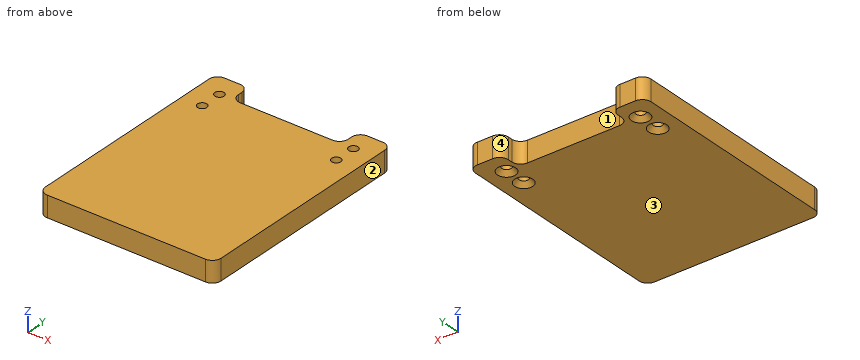
from build123d import *

# Parameters (mm, degrees)
F0_R     = 2.1
F1_DEPTH = 9.525
F2_SIZE2 = 2
F2_SIZE  = 2
F3_W     = 50
F3_H     = 10
F4_DEPTH = 25
F5_R     = 4
F6_R     = 4


with BuildPart() as f1:
    # F0 (on Top) → F1 (new body)
    with BuildSketch(Plane.XY):
        with BuildLine():
            ThreePointArc((40, 47.5), (38.8284271247, 50.3284271247), (36, 51.5))
            Line((36, 51.5), (-36, 51.5))
            ThreePointArc((-36, 51.5), (-38.8284271247, 50.3284271247), (-40, 47.5))
            Line((-40, 47.5), (-40, -47.5))
            ThreePointArc((-40, -47.5), (-38.8284271247, -50.3284271247), (-36, -51.5))
            Line((-36, -51.5), (36, -51.5))
            ThreePointArc((36, -51.5), (38.8284271247, -50.3284271247), (40, -47.5))
            Line((40, -47.5), (40, 47.5))
        make_face()
        with Locations((-30.5, 31.5)):
            Circle(F0_R, mode=Mode.SUBTRACT)
        with Locations((-30.5, 41.5)):
            Circle(F0_R, mode=Mode.SUBTRACT)
        with Locations((30.5, 31.5)):
            Circle(F0_R, mode=Mode.SUBTRACT)
        with Locations((30.5, 41.5)):
            Circle(F0_R, mode=Mode.SUBTRACT)
    extrude(amount=F1_DEPTH)

    # F2
    f2_edges = [f1.edges().sort_by_distance(p)[0] for p in [
        (28.4, 41.5, 0),
        (28.4, 31.5, 0),
        (-32.6, 31.5, 0),
        (-32.6, 41.5, 0),
    ]]
    chamfer(f2_edges, length=F2_SIZE, length2=F2_SIZE2)

    # F3 (on face) → F4 (cut)
    with BuildSketch(Plane.XY.offset(9.525)):
        with Locations((0, 46.5)):
            Rectangle(F3_W, F3_H)
    extrude(amount=-F4_DEPTH, mode=Mode.SUBTRACT)

    # F5
    f5_edges = [f1.edges().sort_by_distance(p)[0] for p in [
        (-25, 51.5, 4.7625),
        (25, 51.5, 4.7625),
    ]]
    fillet(f5_edges, radius=F5_R)

    # F6
    f6_edges = [f1.edges().sort_by_distance(p)[0] for p in [
        (25, 41.5, 4.7625),
        (-25, 41.5, 4.7625),
    ]]
    fillet(f6_edges, radius=F6_R)


solid = f1.part
Model file for the job. Use its own axes, mm. Face numbers are marked on the shaded views. Give positions to 0.01 mm unless a question says otherwise; leave off trailing zeros. Write each loop counter-clockwise with the first axis right and the second up, starting at its lowest first coordinate (ties: lowest second). Pieces come first, ordered by that corner, then holes. Notation, with made-up numbers: M -35.5,39 L 7.5,39 A30 ccw 7.5,69 Z; hole C 74,-32 d5. An arc over 180 degrees is marked long. One line per item, written item: value. Start each with the question number.
Q1. Probe probe 1 along X at (y, z) = (33, 1.5); probe 2 along Y at (x, z) = (30.5, 8.25); probe 3 along Y at (x, z) = (32, 3.5). List the from-to ranges inside material, lowest first. Write a range as [from, to].
Q2. Saw through at A-A, the plane x = -30.5. Write the cut outline in (y, z) (3 decimals).
Q3. Saw through at D-D, the plane x = 8.5. Write the cut outline in (y, z) (3 decimals).
Q4. Drop flat-ended pins along their axis: pin 1 Ø2.5 at (x, y) = (-30.5, 41.5) entering from +Z; pin 2 Ø1.5 at (x, z) = (4.5, 5.5) entering from +Y; pin 3 Ø4 at (x, y) = (4.5, -32) entering from -Z. Give the stop position or say it passes through.
Q5. Saw through at C-C, the plane z = 4.75. Write the cut outline in (x, y).
Q6. Two-plate mould, pull along X, no slides. Class the marked faces 1, 2, 3 and 4: +X half, -X half, draft (parallel to the pull), parting line (faces both ways), or undercut.
Q7. Saw through at B-B, the plane y = 31.5. Write the cut outline in (x, z) (3 decimals), plus the area to 3 significant figures.
Output values:
1. probe 1: x = [-40, -32.62], [-28.38, 28.38], [32.62, 40]
1. probe 2: y = [-51.5, 29.4], [33.6, 39.4], [43.6, 51.5]
1. probe 3: y = [-51.5, 30.03], [32.97, 40.03], [42.97, 51.5]
2. outline: M -51.5,0 L 27.4,0 L 29.4,2 L 29.4,9.525 L -51.5,9.525 Z; M 33.6,2 L 35.6,0 L 37.4,0 L 39.4,2 L 39.4,9.525 L 33.6,9.525 Z; M 43.6,2 L 45.6,0 L 51.5,0 L 51.5,9.525 L 43.6,9.525 Z
3. outline: M -51.5,0 L 41.5,0 L 41.5,9.525 L -51.5,9.525 Z
4. pin 1: passes through
4. pin 2: stops at y = 41.5
4. pin 3: stops at z = 0
5. outline: M -40,-47.5 A4 ccw -36,-51.5 L 36,-51.5 A4 ccw 40,-47.5 L 40,47.5 A4 ccw 36,51.5 L 29,51.5 A4 ccw 25,47.5 L 25,45.5 A4 cw 21,41.5 L -21,41.5 A4 cw -25,45.5 L -25,47.5 A4 ccw -29,51.5 L -36,51.5 A4 ccw -40,47.5 Z; hole C -30.5,31.5 d4.2; hole C -30.5,41.5 d4.2; hole C 30.5,31.5 d4.2; hole C 30.5,41.5 d4.2
6. face 1: undercut
6. face 2: +X half
6. face 3: draft
6. face 4: undercut
7. outline: M -40,0 L -34.6,0 L -32.6,2 L -32.6,9.525 L -40,9.525 Z; M -28.4,2 L -26.4,0 L 26.4,0 L 28.4,2 L 28.4,9.525 L -28.4,9.525 Z; M 32.6,2 L 34.6,0 L 40,0 L 40,9.525 L 32.6,9.525 Z
7. area: 674 mm²
